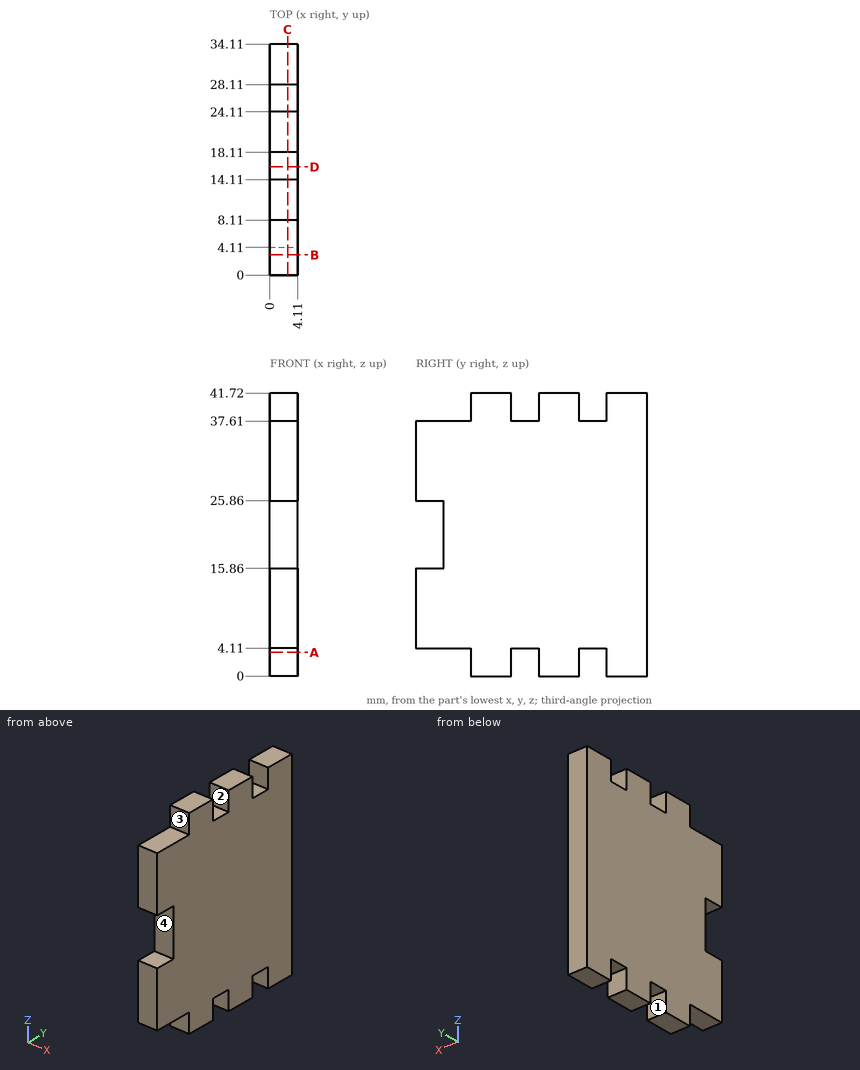
Could you check a few things on this drawing? It's one solid part, dimensions in mm from its lowest x, y, z. A direction names the side the tool comes from. Give positions to 0.01 mm unless a question says otherwise; leave off trailing zeros. Write each loop counter-clockwise with the first axis right and the second up, starting at its lowest first coordinate (ties: lowest second). Pieces come first, ordered by that corner, then holes.
(1) Imagine slicing it at B-B, the plane y = 3. Write out the boundary of the cut face in (x, z).
Output values:
outline: (0, 4.11) - (4.11, 4.11) - (4.11, 15.86) - (0, 15.86) - close; (0, 25.86) - (4.11, 25.86) - (4.11, 37.61) - (0, 37.61) - close
(2) Imagine slicing it at A-A, the plane z = 3.5. Write out the boundary of the cut face in (x, y).
Output values:
outline: (0, 8.11) - (4.11, 8.11) - (4.11, 14.11) - (0, 14.11) - close; (0, 18.11) - (4.11, 18.11) - (4.11, 24.11) - (0, 24.11) - close; (0, 28.11) - (4.11, 28.11) - (4.11, 34.11) - (0, 34.11) - close
(3) Imagine slicing it at D-D, the plane y = 16. Write out the boundary of the cut face in (x, z), and give its area (3 significant figures).
Output values:
outline: (0, 4.11) - (4.11, 4.11) - (4.11, 37.61) - (0, 37.61) - close
area: 138 mm2
(4) Will these pins go through, and if not, where does the flat tip stop? pin 1 (1 mm diameter, centred on x = 3.5, z = 22.5, fed in from -Y); pin 2 (1.2 mm diameter, centred on x = 2.5, z = 39, fed in from -Y); pin 3 (2 mm diameter, centred on x = 2, y = 2.5, fed in from -Z).
Output values:
pin 1: stops at y = 4.11
pin 2: stops at y = 8.11
pin 3: stops at z = 4.11
(5) On a 3-axis mill with a long thin cutter (end or side, diameter ignored), from which of +Z, -Z, +X, -X, +Y, -Y can I reach the whole of each face in a straight line? I mean the marked faces 1, 2, 3 and 4. Say none if no direction works.
Output values:
face 1: -Z, +X, -X
face 2: +Z, +X, -X
face 3: +Z, +X, -X, -Y
face 4: +X, -X, -Y
(6) If I drill on L1, parallel to Z at x = 3.2, y = 3; L2, parallel to Z at x = 3.65, y = 28; L3, parallel to Y at x = 3.8, z = 19, over which ranges is the centre line in solid material (lowest first)?
Output values:
L1: z = 4.11 to 15.86, 25.86 to 37.61
L2: z = 4.11 to 37.61
L3: y = 4.11 to 34.11
(7) Imagine slicing it at C-C, the plane x = 2.6. Write out the boundary of the cut face in (y, z).
Output values:
outline: (0, 4.11) - (8.11, 4.11) - (8.11, 0) - (14.11, 0) - (14.11, 4.11) - (18.11, 4.11) - (18.11, 0) - (24.11, 0) - (24.11, 4.11) - (28.11, 4.11) - (28.11, 0) - (34.11, 0) - (34.11, 41.72) - (28.11, 41.72) - (28.11, 37.61) - (24.11, 37.61) - (24.11, 41.72) - (18.11, 41.72) - (18.11, 37.61) - (14.11, 37.61) - (14.11, 41.72) - (8.11, 41.72) - (8.11, 37.61) - (0, 37.61) - (0, 25.86) - (4.11, 25.86) - (4.11, 15.86) - (0, 15.86) - close
